For this review, take the finished solid that the model builds, in its own axes (mm). Face numbers are marked on the shaded views. A direction names the side the tool comes from. Round coordinates to 2 decimals unless told otherwise and drop trailing zeros. Order: outer loops, then holes, each group sorted by start corner. A loop starts at its lowest first (then second) coordinate and runs counter-clockwise, first axis right, second up. Notation, with made-up numbers: (-25, 2) - (17, 2) arc R25 cw to (17, 17) - close; hole circle Ø2 at (50, 83). An arc over 180 degrees is marked (long way). Write each question's results on one line, items separated by ' | '. Start each with the question number.
(1) For the marked faces 1, 2 and 3, list the 3-axis set-ups (+Z, -Z, +X, -X, +Y, -Y) from which the entire face can be reached by the end or side of a thin tool; tool diameter is ignored.
(2) Take a section at A-A, the plane x = 2.5. Give the boundary of the cut face in (y, z).
(3) Take a section at D-D, the plane z = 45. Give the boundary of the cut face in (x, y), plus the area to 4 significant figures.
(4) For L1, parallel to Y at x = -116.75, z = -2.5; L2, parallel to Y at x = -64, z = 1; L3, parallel to Z at x = 82, y = 0.25, list the stretches that pass through material, from the lowest coordinate up. Write a range as from..to.
(5) Take a section at B-B, the plane x = 67. Give the boundary of the cut face in (y, z).
(6) Insertion check: pin 1 Ø3 at (x, z) = (-7.5, -44.5) entering from -Y; pin 2 Ø0.5 at (x, z) = (-113.5, 2.5) entering from +Y; pin 3 Ø1.5 at (x, y) = (2, -3.5) entering from -Z. Each pin has a flat end and moves straight along its axis. Give the tip position at first contact, or say it passes through.
(7) Take a section at C-C, the plane y = 16.75. Give the boundary of the cut face in (x, z), plus the area to 3 significant figures.
Autodesk Inventor part; units mm, degrees
ref_plane "YZ Plane" through (0, 0, 0) normal (1, 0, 0) x (0, 1, 0)
ref_plane "XZ Plane" through (0, 0, 0) normal (0, 1, 0) x (-1, 0, 0)
ref_plane "XY Plane" through (0, 0, 0) normal (0, 0, 1) x (1, 0, 0)
sketch "Sketch1" plane through (0, 0, 0) normal (0, 1, 0) x (-1, 0, 0)
  line L0 (102.5, 64.5) -> (-102.5, 64.5)
  line L1 (-102.5, 64.5) -> (-102.5, -64.5)
  line L2 (-102.5, -64.5) -> (102.5, -64.5)
  line L3 (102.5, -64.5) -> (102.5, 64.5)
  line L4 (0, 64.5) -> (0, -64.5)
  line L5 (102.5, 0) -> (-102.5, 0)
  point P0 (0, 0)
  dimension "d0" = 129
  dimension "d1" = 205
  dimension "d2" = 0
  dimension "d3" = 0
extrude "Extrusion1" add sketch "Sketch1" along normal blind 5
sketch "Sketch2" plane through (0, 5, 0) normal (0, 1, 0) x (1, 0, 0)
  circle A0 centre (2.5, 2.5) radius 4.5
  circle A1 centre (2.5, 2.5) radius 6
  circle A2 centre (2.5, 2.5) radius 7.5
  circle A3 centre (2.5, 2.5) radius 2.35
  line L0 (6.8875, 3.5) -> (9.933, 3.5)
  line L1 (6.8875, 1.5) -> (9.933, 1.5)
  line L2 (-102.5, 64.5) -> (-102.5, -64.5)
  line L3 (102.5, -64.5) -> (102.5, 64.5)
  line L4 (-102.5, -64.5) -> (102.5, -64.5)
  line L5 (102.5, -64.5) -> (102.5, 64.5)
  line L6 (102.5, 64.5) -> (-102.5, 64.5)
  line L7 (-102.5, 64.5) -> (-102.5, -64.5)
  line L8 (-102.5, -64.5) -> (102.5, -64.5)
  point P0 (0, -64.5)
  point P1 (8.4161, 3.5)
  point P2 (8.4161, 1.5)
  point P3 (-102.5, 0)
  dimension "d18" = 9
  dimension "d19" = 12
  dimension "d20" = 15
  dimension "d21" = 4.7
  dimension "d22" = 1
  dimension "d23" = 1
  dimension "d26" = 0
  dimension "d40" = 67
  dimension "d41" = 105
extrude "Extrusion2" add sketch "Sketch2" along normal blind 20 contours A0 L1 A1 L0 | L0 A2 L1 A1 | A1 L1 A2 L0 picked at (-2.8948, 1.6483)
sketch "Sketch3" plane through (-102.5, 0, 64.5) normal (0, 0, 1) x (1, 0, 0)
  circle A0 centre (105, 2.5) radius 4.5
  circle A1 centre (105, 2.5) radius 6
  circle A2 centre (105, 2.5) radius 7.5
  circle A3 centre (105, 2.5) radius 2.35
  line L0 (109.3875, 3.5) -> (112.433, 3.5)
  line L1 (109.3875, 1.5) -> (112.433, 1.5)
  line L2 (0, 0) -> (0, 5)
  point P0 (102.5, 0)
  point P1 (0, 2.5)
  point P2 (110.9161, 3.5)
  point P3 (110.9161, 1.5)
  dimension "d30" = 9
  dimension "d31" = 12
  dimension "d32" = 15
  dimension "d33" = 4.7
  dimension "d34" = 1
  dimension "d35" = 1
  dimension "d36" = 0
  dimension "d37" = 105
  dimension "d38" = 0
extrude "Extrusion3" add sketch "Sketch3" along normal blind 20 and the other way blind 5 contours A0 L1 A1 L0 | L0 A2 L1 A1 | A1 L1 A2 L0 picked at (99.6052, 1.6483)
sketch "Sketch4" plane through (-102.5, 0, -64.5) normal (-1, 0, 0) x (0, 0, 1)
  circle A0 centre (62, 2.5) radius 4.5
  circle A1 centre (62, 2.5) radius 6
  circle A2 centre (62, 2.5) radius 7.5
  circle A3 centre (62, 2.5) radius 2.35
  line L0 (66.3875, 3.5) -> (69.433, 3.5)
  line L1 (66.3875, 1.5) -> (69.433, 1.5)
  line L2 (129, 0) -> (129, 5)
  point P0 (64.5, 0)
  point P1 (129, 2.5)
  point P2 (67.9161, 3.5)
  point P3 (67.9161, 1.5)
  dimension "d46" = 9
  dimension "d47" = 12
  dimension "d48" = 15
  dimension "d49" = 4.7
  dimension "d50" = 1
  dimension "d51" = 1
  dimension "d52" = 0
  dimension "d53" = 0
  dimension "d54" = 67
extrude "Extrusion4" add sketch "Sketch4" along normal blind 20 and the other way blind 5 contours A0 L1 A1 L0 | L0 A2 L1 A1 | A1 L1 A2 L0 picked at (56.6052, 1.6483)
properties part number "GroundCorrected"
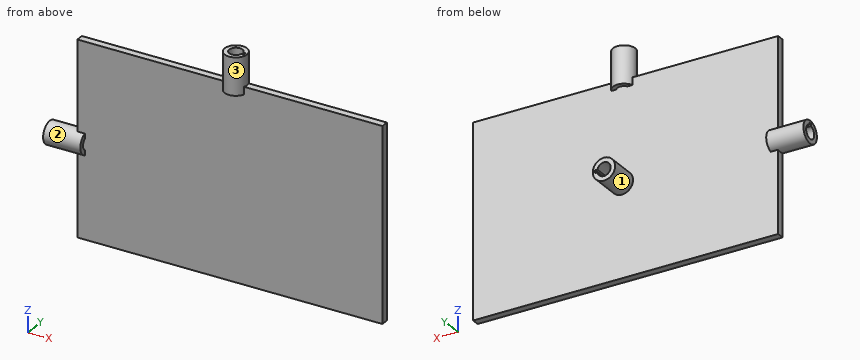
Results below:
1) face 1: +Y | face 2: -X | face 3: +Z
2) outline: (-5, 59.5) - (-2, 59.5) - (-2, 84.5) - (-5, 84.5) - close; (0, -64.5) - (5, -64.5) - (5, -10) - (25, -10) - (25, -7) - (5, -7) - (5, 2) - (25, 2) - (25, 5) - (5, 5) - (5, 64.5) - (0, 64.5) - close; (7, 59.5) - (10, 59.5) - (10, 84.5) - (7, 84.5) - close
3) outline: (-102.5, 0) - (102.5, 0) - (102.5, 5) - (-102.5, 5) - close | area: 1,025 mm^2
4) L1: y = -5..-2, 7..10 | L2: y = 0..5 | L3: z = -64.5..64.5
5) outline: (0, -64.5) - (5, -64.5) - (5, 64.5) - (0, 64.5) - close
6) pin 1: stops at y = 0 | pin 2: stops at y = 8.3 | pin 3: stops at z = 59.5
7) outline: circle Ø15 at (2.5, -2.5); hole (6.89, -3.5) - (8.42, -3.5) arc R6 ccw to (8.42, -1.5) - (6.89, -1.5) arc R4.5 ccw (long way) to start | area: 110 mm^2
